Read the model definition and answer for the solid it produces. Units are mm, in the model's axes. A direction names the side the tool comes from. Give positions to 0.01 mm unless a question says otherwise; leave off trailing zeros. Write each loop counter-clockwise with the first axis right and the second up, starting at its lowest first coordinate (ties: lowest second). Pieces come first, ordered by that corner, then holes. Notation, with made-up numbers: (-21, -21) - (-4, -21) arc R28 cw to (-4, 4) - close; hole circle Ø7 at (78.5, -31). An arc over 180 degrees is marked (long way). Answer as a JSON object with one key per item and string values. Group by question number.
```python
from build123d import *

# Parameters (mm, degrees)
SKETCH1_W           = 12
SKETCH1_H           = 16
SKETCH1_R           = 2.1
SKETCH1_W_2         = 2
BOSS_EXTRUDE1_DEPTH = 20
FILLET1_R           = 5
SKETCH2_W           = 9
SKETCH2_H           = 1.9
BOSS_EXTRUDE2_DEPTH = 5
SKETCH4_W           = 12
SKETCH4_H           = 20
BOSS_EXTRUDE3_DEPTH = 18.5
FILLET2_R           = 5.1
SKETCH5_W           = 17.4
SKETCH5_H           = 12
BOSS_EXTRUDE4_DEPTH = 8
BOSS_EXTRUDE5_DEPTH = 15
FILLET4_R           = 5
FILLET5_R           = 2


with BuildPart() as part:
    # Sketch1 → Boss-Extrude1 (new body)
    # profile 1 of 2: a face of its own
    with BuildSketch(Plane(origin=(0, 0, 0), x_dir=(1, 0, 0), z_dir=(0, 1, 0))):
        Rectangle(SKETCH1_W, SKETCH1_H)
        with Locations(Location((0, 0, 0), (0, 0, 270))):
            Circle(SKETCH1_R, mode=Mode.SUBTRACT)
    # profile 2 of 2: a face of its own
    with BuildSketch(Plane(origin=(0, 0, 0), x_dir=(1, 0, 0), z_dir=(0, 1, 0))):
        with Locations((7, 0)):
            Rectangle(SKETCH1_W_2, SKETCH1_H)
    extrude(amount=BOSS_EXTRUDE1_DEPTH)

    # Fillet1
    fillet1_edges = [part.edges().sort_by_distance(p)[0] for p in [
        (-6, 10, 8),
        (-6, 10, -8),
    ]]
    fillet(fillet1_edges, radius=FILLET1_R)

    # Sketch2 → Boss-Extrude2 (add)
    with BuildSketch(Plane(origin=(0, 20, 0), x_dir=(1, 0, 0), z_dir=(0, 1, 0))):
        with Locations((3.5, 7.05)):
            Rectangle(SKETCH2_W, SKETCH2_H)
        with Locations((3.5, -7.05)):
            Rectangle(SKETCH2_W, SKETCH2_H)
    extrude(amount=BOSS_EXTRUDE2_DEPTH)

    # Sketch4 → Boss-Extrude3 (add)
    with BuildSketch(Plane(origin=(8, 0, 0), x_dir=(0, 0, -1), z_dir=(1, 0, 0))):
        with Locations((0, 10)):
            Rectangle(SKETCH4_W, SKETCH4_H)
    extrude(amount=BOSS_EXTRUDE3_DEPTH)

    # Fillet2
    fillet2_edges = [part.edges().sort_by_distance(p)[0] for p in [
        (26.5, 20, 0),
    ]]
    fillet(fillet2_edges, radius=FILLET2_R)

    # Sketch5 → Boss-Extrude4 (add)
    with BuildSketch(Plane.XZ):
        with Locations((17.8, 0)):
            Rectangle(SKETCH5_W, SKETCH5_H)
    extrude(amount=BOSS_EXTRUDE4_DEPTH)

    # Sketch8 → Boss-Extrude5 (add)
    with BuildSketch(Plane(origin=(26.5, 0, 0), x_dir=(0, 0, -1), z_dir=(1, 0, 0))):
        Polygon((-6, -8), (-6, -0.5), (6, 0.128893351), (6, -8), align=None)
    extrude(amount=BOSS_EXTRUDE5_DEPTH)

    # Fillet4
    fillet4_edges = [part.edges().sort_by_distance(p)[0] for p in [
        (41.5, -8, 0),
    ]]
    fillet(fillet4_edges, radius=FILLET4_R)

    # Fillet5
    fillet5_edges = [part.edges().sort_by_distance(p)[0] for p in [
        (8, 10, 6),
    ]]
    fillet(fillet5_edges, radius=FILLET5_R - 0.0001)  # a hair under: the kernel refuses the full size
    fillet5_2_edges = [part.edges().sort_by_distance(p)[0] for p in [
        (8, 10, -6),
    ]]
    fillet(fillet5_2_edges, radius=FILLET5_R - 0.0001)  # a hair under: the kernel refuses the full size
    fillet5_3_edges = [part.edges().sort_by_distance(p)[0] for p in [
        (-1, 20, -7.05),
    ]]
    fillet(fillet5_3_edges, radius=FILLET5_R)
    fillet5_4_edges = [part.edges().sort_by_distance(p)[0] for p in [
        (-1, 20, 7.05),
    ]]
    fillet(fillet5_4_edges, radius=FILLET5_R)


solid = part.part
```
1) For a pull along Z with two mould halves and no side action, classify faces 5 (the flat face through (22, 3, -6)), 6 (the cylindrical face through (0.631, 9.86, 2.003)), 7 (the cylindrical face through (24.966, 18.546, -0.084)) as released by +Z, released by -Z, zero draft, split by the parting line, or undercut.
2) A flat-ended cylindrical pin translates along its axis: pin 1 Ø8 at (x, y) = (34, 1.5) entering from -Z. Find the tip coordinate at first contact, or state that the pin passes through.
3) Find section B-B, the plane x = 16. Write down the section's boundary in (y, z), and give its area (3 significant figures).
4) Find section A-A, the plane y = -2.5. Write down the section's boundary in (x, z).
5) Which of the six approach directions +Z, -Z, +X, -X, +Y, -Y give full straight-line access (tool end or side, diameter ignored) to faces 1 (the flat face through (22, 3, 6)), 2 (the flat face through (-1, 23, 7)), 3 (the flat face through (23, -8, 0)), 4 (the flat face through (33.89, -0.19, 0.08))?
Values follow:
{
 "1": {"face 5": "released by -Z", "face 6": "undercut", "face 7": "zero draft"},
 "2": {"pin 1": "stops at z = -6"},
 "3": {"outline": "(-8, -6) - (20, -6) - (20, 6) - (-8, 6) - close", "area": "336 mm2"},
 "4": {"outline": "(9.1, -6.21) arc R2 cw to (10, -6) - (41.5, -6) - (41.5, 6) - (10, 6) arc R2 cw to (9.1, 6.21) - close"},
 "5": {"face 1": "+Z, +X, +Y, -Y", "face 2": "+Z, -Z, -X, +Y", "face 3": "+Z, -Z, +X, -X, -Y", "face 4": "+Z, +X, +Y"}
}
